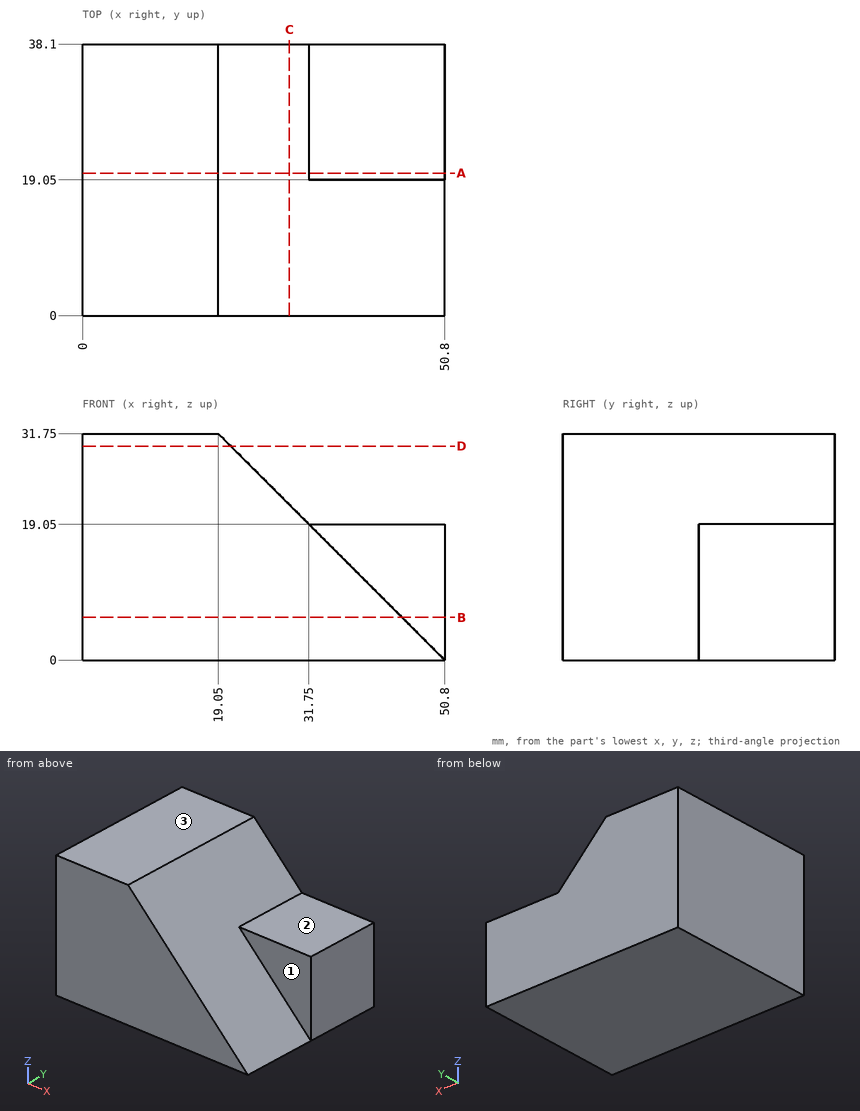
Verification items for this drawing (mm, ordinates from the low corner). A direction names the side the tool comes from. Coordinates: 2 decimals unless noted, no trailing zeros. Loops run counter-clockwise (first coordinate to the right, second up) from the corner with the lowest first, then second, coordinate; pieces in that order, holes last. Notation, with made-up numbers: (-19, -13.5) -> (5, -13.5) arc R13 cw to (5, -9.5) -> close; hole circle Ø5 at (6.5, 44.5). An arc over 180 degrees is marked (long way). Answer in a Markdown table with one row per item. Add a question column.
1. Section check A-A, the plane y = 20. Enter the section's corners in (x, z).
2. Section check B-B, the plane z = 6. Enter the section's corners in (x, y).
3. Access from +Z, -Z, +X, -X, +Y, -Y to the whole of each face (thin tool, end or side, straight path). Record for the marked faces 1, 2 and 3.
4. Material ranges on probe 1 along Z at (x, y) = (45, 31); probe 2 along X at (y, z) = (5, 25); probe 3 along X at (y, z) = (6, 6.5), recorded low to high. Write a range as [from, to].
5. Depth check by flat-ended pin: P1, Ø15, axis at x = 44, y = 33, coming from the +Z side. Enter the tip coordinate at first touch or a pass-through.
6. Section check C-C, the plane x = 29. Enter the section's corners in (y, z), then the cut area to 3 significant figures.
7. Section check D-D, the plane z = 30. Enter the section's corners in (x, y), then the cut area to 3 significant figures.
Derived:
| question | item | result |
|---|---|---|
| 1 | outline | (0, 0) -> (50.8, 0) -> (50.8, 19.05) -> (31.75, 19.05) -> (19.05, 31.75) -> (0, 31.75) -> close |
| 2 | outline | (0, 0) -> (44.8, 0) -> (44.8, 19.05) -> (50.8, 19.05) -> (50.8, 38.1) -> (0, 38.1) -> close |
| 3 | face 1 | +Z, +X, -Y |
| 3 | face 2 | +Z, +X, +Y, -Y |
| 3 | face 3 | +Z, +X, -X, +Y, -Y |
| 4 | probe 1 | z = [0, 19.05] |
| 4 | probe 2 | x = [0, 25.8] |
| 4 | probe 3 | x = [0, 44.3] |
| 5 | P1 | stops at z = 19.05 |
| 6 | outline | (0, 0) -> (38.1, 0) -> (38.1, 21.8) -> (0, 21.8) -> close |
| 6 | area | 831 mm² |
| 7 | outline | (0, 0) -> (20.8, 0) -> (20.8, 38.1) -> (0, 38.1) -> close |
| 7 | area | 792 mm² |
